```python
from build123d import *

# Parameters (mm, degrees)
SKETCH1_W           = 3.22
SKETCH1_H           = 41.98
BOSS_EXTRUDE1_DEPTH = 4.98
CUT_EXTRUDE1_DEPTH  = 41.98
FILLET1_R           = 0.6
FILLET2_R           = 0.3
SKETCH4_R           = 0.6
SKETCH4_R_2         = 0.2
SKETCH4_R_3         = 0.28
SKETCH4_R_4         = 0.36
SKETCH4_R_5         = 0.44
SKETCH4_R_6         = 0.52
CUT_EXTRUDE2_DEPTH  = 4.98


with BuildPart() as part:
    # Sketch1 → Boss-Extrude1 (new body)
    with BuildSketch(Plane(origin=(0, 0, 0), x_dir=(1, 0, 0), z_dir=(0, 1, 0))):
        with Locations((1.61, -20.99)):
            Rectangle(SKETCH1_W, SKETCH1_H)
    extrude(amount=BOSS_EXTRUDE1_DEPTH)

    # Sketch2 → Cut-Extrude1 (cut)
    with BuildSketch(Plane.XY.offset(41.98)):
        Polygon((0, 4.98), (3.22, 4.98), (3.22, 3.78), align=None)
    extrude(amount=-CUT_EXTRUDE1_DEPTH, mode=Mode.SUBTRACT)

    # Fillet1
    fillet1_edges = [part.edges().sort_by_distance(p)[0] for p in [
        (3.22, 3.78, 20.99),
        (1.61, 4.38, 41.98),
        (1.61, 4.38, 0),
    ]]
    fillet(fillet1_edges, radius=FILLET1_R)

    # Fillet2
    # the kernel refuses this fillet: 0.3 mm, written as the material it takes off along each edge
    with BuildSketch(Plane(origin=(0, 4.98, 42.459891752), x_dir=(0, -1, 0), z_dir=(0, 0, -1))) as fillet2_piece_1:
        with BuildLine():
            CenterArc((FILLET2_R * 1.43985566994, -FILLET2_R), FILLET2_R, 90, 110.438955915)
            Line((FILLET2_R * 0.50281089434, -FILLET2_R * 1.34920923314), (0, 0))
            Line((0, 0), (FILLET2_R * 1.43985566994, 0))
        make_face()
    extrude(amount=42.939783505, mode=Mode.SUBTRACT)

    # Sketch4 → Cut-Extrude2 (cut)
    with BuildSketch(Plane(origin=(-1.629578944, 0.607296501, 0), x_dir=(0, 0, 1), z_dir=(-0.9370447756039936, 0.3492092331443447, 0))):
        with Locations((3.365, 4.666482983)):
            Circle(SKETCH4_R)
        with Locations((38.615, 4.666482983)):
            Circle(SKETCH4_R_2)
        with Locations((31.565, 4.666482983)):
            Circle(SKETCH4_R_3)
        with Locations((24.515, 4.666482983)):
            Circle(SKETCH4_R_4)
        with Locations((17.465, 4.666482983)):
            Circle(SKETCH4_R_5)
        with Locations((10.415, 4.666482983)):
            Circle(SKETCH4_R_6)
    extrude(amount=-CUT_EXTRUDE2_DEPTH, mode=Mode.SUBTRACT)


solid = part.part
```
Geometry: final body of the model. Coordinates: model frame, mm. Coordinates: 2 decimals unless noted, no trailing zeros. Order: outer loops, then holes, each group sorted by start corner. A loop starts at its lowest first (then second) coordinate and runs counter-clockwise, first axis right, second up. Notation, with made-up numbers: (81, -40) -> (132, -40) arc R24 ccw to (132, -14) -> close; hole circle Ø6 at (17.25, 56). An arc over 180 degrees is marked (long way). Use CSV: the item, a comma, the result in double quotes.
1) Section A-A on z = 14.5. Output: boundary loops of the cut face in (x, y), then the cut area to 3 significant figures.
Findings:
outline,"(0, 0) -> (3.22, 0) -> (3.22, 3.36) arc R0.6 ccw to (2.83, 3.93) -> (0.4, 4.83) arc R0.3 ccw to (0, 4.55) -> close"
area,"14.0 mm^2"
2) Mould query, pull axis Z, two halves, no side actions, for faces 1 (the flat face through (1.634, 4.371, 40.115)), 2 (the cylindrical face through (1.6, 4, 24.5)), 3 (the cylindrical face through (1.688, 4.158, 41.809)). Classes: +Z half, -Z half, draft (parallel to the pull), parting line (faces both ways), or undercut.
Findings:
face 1,"draft"
face 2,"undercut"
face 3,"+Z half"
3) Line query: line 1 (Y direction, x = 2.85, z = 16.5); line 2 (X direction, y = 3.6, z = 35); line 3 (Y direction, x = 3, z = 26). Output: solid intervals per line, ascending.
Findings:
line 1,"y = 0 to 3.92"
line 2,"x = 0 to 3.17"
line 3,"y = 0 to 3.83"
